Read the model definition and answer for the solid it produces. Units are mm, in the model's axes. A direction names the side the tool comes from. Coordinates: 2 decimals unless noted, no trailing zeros. Write each loop counter-clockwise with the first axis right and the second up, starting at its lowest first coordinate (ties: lowest second). Pieces come first, ordered by that corner, then holes. Notation, with made-up numbers: (-24, 54.25) -> (29, 54.25) arc R26 ccw to (29, 87.25) -> close; hole circle Ø6 at (62.5, 61). An arc over 180 degrees is marked (long way). Return JSON: item names as keys, results as strings.
from build123d import *

# Parameters (mm, degrees)
F0_W     = 100
F0_H     = 50
F1_DEPTH = 25
F2_W     = 10
F2_H     = 10
F3_DEPTH = 15
F4_DEPTH = 18


with BuildPart() as f1:
    # F0 (on Front) → F1 (new body)
    with BuildSketch(Plane.XZ):
        with Locations((-18.900802, 25)):
            Rectangle(F0_W, F0_H)
    extrude(amount=F1_DEPTH)

    # F2 (on face) → F3 (join)
    with BuildSketch(Plane.XZ.offset(25)):
        with Locations((-63.900802, 5)):
            Rectangle(F2_W, F2_H)
        with Locations((-63.900802, 45)):
            Rectangle(F2_W, F2_H)
        with Locations((26.099198, 45)):
            Rectangle(F2_W, F2_H)
        with Locations((26.099198, 5)):
            Rectangle(F2_W, F2_H)
    extrude(amount=F3_DEPTH)

    # F1_face (on face) → F4 (cut)
    with BuildSketch(Plane(origin=(-18.900802, -25, 25), x_dir=(1, 0, 0), z_dir=(0, -1, 0))):
        Polygon((40, 15), (40, 25), (-40, 25), (-40, 15), (-50, 15), (-50, -15), (-40, -15), (-40, -25), (40, -25), (40, -15), (50, -15), (50, 15), align=None)
    extrude(amount=-F4_DEPTH, mode=Mode.SUBTRACT)


solid = f1.part
1. A tool of negligible diameter and unlimited length cuts with its end or side. For faces 4 (the face through (-58.901, -24, 5)), 5 (the face through (-64, -23, 40)), 6 (the face through (26, -40, 5)), from which of +Z, -Z, +X, -X, +Y, -Y can it reach the whole face along a straight path? Write none if from no direction.
Taken from the geometry:
{"face 4": "+Z, -Z, -Y", "face 5": "+X, -X, -Y", "face 6": "+Z, -Z, +X, -X, -Y"}
2. For a pull along Z with two mould halves and no side action, classify faces 1 (the face through (-20, -6, 0)), 2 (the face through (26, -40, 45)), 3 (the face through (-20, -7, 25)) as +Z half, -Z half, draft (parallel to the pull), parting line (faces both ways), or undercut.
Taken from the geometry:
{"face 1": "-Z half", "face 2": "draft", "face 3": "undercut"}
3. Consider L1, parallel to X at y = -33, z = 48; L2, parallel to Z at x = -60, y = -26; L3, parallel to Y at x = -37, z = 4. Determine where each line is inside the solid, lowest interval first.
Taken from the geometry:
{"L1": "x = -68.9 to -58.9, 21.1 to 31.1", "L2": "z = 0 to 10, 40 to 50", "L3": "y = -7 to 0"}
4. The part is cut by section C-C (x = -44). Determine the outline of the cut face in (y, z).
Taken from the geometry:
{"outline": "(-7, 0) -> (0, 0) -> (0, 50) -> (-7, 50) -> close"}
5. The part is cut by section D-D (z = 36.5). Determine the outline of the cut face in (x, y).
Taken from the geometry:
{"outline": "(-68.9, -7) -> (31.1, -7) -> (31.1, 0) -> (-68.9, 0) -> close"}
6. The part is cut by section B-B (z = 42). Determine the outline of the cut face in (x, y).
Taken from the geometry:
{"outline": "(-68.9, -40) -> (-58.9, -40) -> (-58.9, -7) -> (21.1, -7) -> (21.1, -40) -> (31.1, -40) -> (31.1, 0) -> (-68.9, 0) -> close"}
7. The part is cut by section A-A (y = -28.5). Determine the outline of the cut face in (x, z), then the cut area to 3 significant figures.
Taken from the geometry:
{"outline": "(-68.9, 0) -> (-58.9, 0) -> (-58.9, 10) -> (-68.9, 10) -> close; (-68.9, 40) -> (-58.9, 40) -> (-58.9, 50) -> (-68.9, 50) -> close; (21.1, 0) -> (31.1, 0) -> (31.1, 10) -> (21.1, 10) -> close; (21.1, 40) -> (31.1, 40) -> (31.1, 50) -> (21.1, 50) -> close", "area": "400 mm2"}
8. Flat-ended cylindrical pins translate along their axes: pin 1 Ø12 at (x, y) = (-50, -19.5) entering from -Z; pin 2 Ø3 at (x, y) = (-62, -27.5) entering from -Z; pin 3 Ø25 at (x, z) = (5.5, 12.5) entering from -Y. Find the tip coordinate at first contact, or state that the pin passes through.
Taken from the geometry:
{"pin 1": "passes through", "pin 2": "stops at z = 0", "pin 3": "stops at y = -7"}
